from build123d import *

# Parameters (mm, degrees)
SKETCH_R     = 4.95
PAD_DEPTH    = 7.1
SKETCH001_R  = 0.5
PAD001_DEPTH = 5
SKETCH002_R  = 3
POCKET_DEPTH = 0.4


with BuildPart() as part:
    # Sketch → Pad (new body)
    with BuildSketch(Plane.XY):
        Circle(SKETCH_R)
    extrude(amount=PAD_DEPTH)

    # Sketch001 → Pad001 (new body)
    with BuildSketch(Plane(origin=(0, 0, 0), x_dir=(1, 0, 0), z_dir=(0, 0, -1))):
        with Locations((2.5, 0)):
            Circle(SKETCH001_R)
        with Locations((-2.5, 0)):
            Circle(SKETCH001_R)
    extrude(amount=PAD001_DEPTH)

    # Sketch002 → Pocket (cut)
    with BuildSketch(Plane.XY.offset(7.1)):
        Circle(SKETCH002_R)
    extrude(amount=-POCKET_DEPTH, mode=Mode.SUBTRACT)


solid = part.part
The model under review builds one solid part; all positions refer to its coordinate system, in mm. A direction names the side the tool comes from. Coordinates: 2 decimals unless noted, no trailing zeros. Order: outer loops, then holes, each group sorted by start corner. A loop starts at its lowest first (then second) coordinate and runs counter-clockwise, first axis right, second up. Notation, with made-up numbers: (31, -8.75) -> (57, -8.75) arc R18 ccw to (57, 17.25) -> close; hole circle Ø3 at (84, -10.5). An arc over 180 degrees is marked (long way). Answer in a Markdown table with one row per item.
(1) Wall thickness on line 1 along Y through (x, z) = (0, 6.9); line 2 along X through (y, z) = (0, -3.5); line 3 along Y through (x, z) = (-2.5, -0.75): over which ranges is each line inside the solid? List them lowest first.
Answers:
| item | result |
|---|---|
| line 1 | -4.95 to -3, 3 to 4.95 |
| line 2 | -3 to -2, 2 to 3 |
| line 3 | -0.5 to 0.5 |
(2) Machinability: for faces 1 (the cylindrical face through (-3, 0, -2)), 2 (the flat face through (-2.5, 0, -5)), 3 (the cylindrical face through (-3, 0.1, 6.9)), which of the approach directions +Z, -Z, +X, -X, +Y, -Y give a long, thin tool a straight path to every point of the face, cutting with its end or side? Answer none if there is none.
Answers:
| item | result |
|---|---|
| face 1 | -Z |
| face 2 | -Z, +X, -X, +Y, -Y |
| face 3 | +Z |
(3) Insertion check: pin 1 (1.8 mm diameter, centred on x = -1.5, y = 0, fed in from +Z); pin 2 (2 mm diameter, centred on y = 0, z = -3.5, fed in from +X); pin 3 (2 mm diameter, centred on y = 1, z = -3, fed in from -X). Each pin has a flat end and moves straight along its axis. Give the tip position at first contact, or say it passes through.
Answers:
| item | result |
|---|---|
| pin 1 | z = 6.7 |
| pin 2 | x = 3 |
| pin 3 | x = -3 |
(4) Consider section C-C (y = 0). Write out the cut boundary in (x, z).
Answers:
| item | result |
|---|---|
| outline | (-4.95, 0) -> (-3, 0) -> (-3, -5) -> (-2, -5) -> (-2, 0) -> (2, 0) -> (2, -5) -> (3, -5) -> (3, 0) -> (4.95, 0) -> (4.95, 7.1) -> (3, 7.1) -> (3, 6.7) -> (-3, 6.7) -> (-3, 7.1) -> (-4.95, 7.1) -> close |
(5) Consider section B-B (z = -2.5). Write out the cut boundary in (x, y).
Answers:
| item | result |
|---|---|
| outline | circle Ø1 at (-2.5, 0); circle Ø1 at (2.5, 0) |
(6) Consider section D-D (z = 5.5). Write out the cut boundary in (x, y).
Answers:
| item | result |
|---|---|
| outline | circle Ø9.9 at (0, 0) |
(7) The part is to be moulded in two halves that separate along Y. For faces 4 (the flat face through (0, 0, 6.7)), 5 (the flat face through (3.2, 0.1, 7.1)), 6 (the cylindrical face through (4.72, 1.49, 3.5)), say which applies: +Y half, -Y half, draft (parallel to the pull), parting line (faces both ways), or undercut.
Answers:
| item | result |
|---|---|
| face 4 | undercut |
| face 5 | draft |
| face 6 | parting line |
(8) Consider section A-A (x = 0). Write out the cut boundary in (y, z), plus the area to 3 significant figures.
Answers:
| item | result |
|---|---|
| outline | (-4.95, 0) -> (4.95, 0) -> (4.95, 7.1) -> (3, 7.1) -> (3, 6.7) -> (-3, 6.7) -> (-3, 7.1) -> (-4.95, 7.1) -> close |
| area | 67.9 mm² |
